Build history of the part. All positions in model axes, mm. A direction names the side the tool comes from. Coordinates: 2 decimals unless noted, no trailing zeros. Loops run counter-clockwise (first coordinate to the right, second up) from the corner with the lowest first, then second, coordinate; pieces in that order, holes last. Notation, with made-up numbers: (79, 56) - (108, 56) arc R29 cw to (108, 77) - close; hole circle Ø1 at (-35, 8). An arc over 180 degrees is marked (long way). One line per item, written item: value.
```python
from build123d import *

# Parameters (mm, degrees)
BOSS_EXTRUDE1_DEPTH = 80
BOSS_EXTRUDE2_DEPTH = 17
SKETCH3_R           = 7.5
CUT_EXTRUDE1_DEPTH  = 17
CUT_EXTRUDE2_DEPTH  = 70
SKETCH6_R           = 6
CUT_EXTRUDE3_DEPTH  = 20


with BuildPart() as part:
    # Sketch1 → Boss-Extrude1 (new body)
    with BuildSketch(Plane.XY):
        Polygon((-12, 17), (-12, -17), (29, -17), (29, -30), (-29, -30), (-29, 30), (29, 30), (29, 17), align=None)
    extrude(amount=-BOSS_EXTRUDE1_DEPTH)

    # Sketch2 → Boss-Extrude2 (add)
    with BuildSketch(Plane.ZY.offset(29)):
        with BuildLine():
            Line((-70, 70.5), (-70, 35.68393157))
            ThreePointArc((-70, 35.68393157), (-71.664785013, 31.664785013), (-75.68393157, 30))
            Line((-75.68393157, 30), (-4.31606843, 30))
            ThreePointArc((-4.31606843, 30), (-8.335214987, 31.664785013), (-10, 35.68393157))
            Line((-10, 35.68393157), (-10, 70.5))
            ThreePointArc((-10, 70.5), (-40, 100.5), (-70, 70.5))
        make_face()
    extrude(amount=-BOSS_EXTRUDE2_DEPTH)

    # Sketch3 → Cut-Extrude1 (cut)
    with BuildSketch(Plane.ZY.offset(29)):
        with Locations(Location((-40, 70.5, 0), (0, 0, 270))):
            Circle(SKETCH3_R)
    extrude(amount=-CUT_EXTRUDE1_DEPTH, mode=Mode.SUBTRACT)

    # Sketch4 → Cut-Extrude2 (cut)
    with BuildSketch(Plane(origin=(0, 30, 0), x_dir=(1, 0, 0), z_dir=(0, 1, 0))):
        with BuildLine():
            Line((9.5, 66), (9.5, 14))
            ThreePointArc((9.5, 14), (16, 7.5), (22.5, 14))
            Line((22.5, 14), (22.5, 66))
            ThreePointArc((22.5, 66), (16, 72.5), (9.5, 66))
        make_face()
    extrude(amount=-CUT_EXTRUDE2_DEPTH, mode=Mode.SUBTRACT)

    # Sketch6 → Cut-Extrude3 (cut)
    with BuildSketch(Plane(origin=(-12, 0, 0), x_dir=(0, 0, -1), z_dir=(1, 0, 0))):
        with Locations(Location((18.5, 0, 0), (0, 0, 90))):
            Circle(SKETCH6_R)
        with Locations(Location((61.5, 0, 0), (0, 0, 90))):
            Circle(SKETCH6_R)
    extrude(amount=-CUT_EXTRUDE3_DEPTH, mode=Mode.SUBTRACT)


solid = part.part
```
Item 1: Cut at D-D, the plane x = -16. Write the cut outline in (y, z).
Check result:
outline: (-30, -80) - (30, -80) - (30, -75.68) arc R5.68 cw to (35.68, -70) - (70.5, -70) arc R30 ccw to (70.5, -10) - (35.68, -10) arc R5.68 cw to (30, -4.32) - (30, 0) - (-30, 0) - close; hole circle Ø12 at (0, -61.5); hole circle Ø12 at (0, -18.5); hole circle Ø15 at (70.5, -40)
Item 2: Cut at A-A, the plane z = -40. Write the cut outline in (x, y).
Check result:
outline: (-29, -30) - (9.5, -30) - (9.5, -17) - (-12, -17) - (-12, 17) - (9.5, 17) - (9.5, 30) - (-12, 30) - (-12, 63) - (-29, 63) - close; (-29, 78) - (-12, 78) - (-12, 100.5) - (-29, 100.5) - close; (22.5, -30) - (29, -30) - (29, -17) - (22.5, -17) - close; (22.5, 17) - (29, 17) - (29, 30) - (22.5, 30) - close
Item 3: Drop flat-ended pins along their axis: P1, Ø24, axis at y = 70.5, z = -40, coming from the -X side; P2, Ø12.5, axis at x = 5, z = -44.5, coming from the +Y side; P3, Ø12, axis at x = -10, y = 61.5, coming from the -Z side; P4, Ø13.5, axis at x = -18, y = 48.5, coming from the +Z side. Give the stop position or say it passes through.
Check result:
P1: stops at x = -29
P2: stops at y = 30
P3: stops at z = -70
P4: stops at z = -10
Item 4: Cut at B-B, the plane x = 13.5. Write the cut outline in (y, z).
Check result:
outline: (-30, -80) - (-17, -80) - (-17, -72) - (-30, -72) - close; (-30, -8) - (-17, -8) - (-17, 0) - (-30, 0) - close; (17, -80) - (30, -80) - (30, -72) - (17, -72) - close; (17, -8) - (30, -8) - (30, 0) - (17, 0) - close
Item 5: Pull direction Y, two halves, no side cores. Call faces 4 (the face through (29, -23, -39)), 5 (the face through (4, 17, -39)), 6 (the face through (-20.381, 5.723, -59.698)), 7 (the face through (-20.62, 31.71, -71.62)): released by +Y, released by -Y, zero draft, split by the parting line, or undercut.
Check result:
face 4: zero draft
face 5: undercut
face 6: undercut
face 7: released by +Y
Item 6: Tool access for faces 1 (the face through (15.9, 23.6, -7.5)), 2 (the face through (-12, 58, -40)), 3 (the face through (-21, 53, -70)): list every direction of +Z, -Z, +X, -X, +Y, -Y with a clear straight run to the whole face (end or side of a thin tool).
Check result:
face 1: +Y, -Y
face 2: +Z, -Z, +X, +Y
face 3: -Z, +X, -X, +Y
Item 7: Probe probe 1 along Z at (x, y) = (-18.5, 0); probe 2 along Y at (x, z) = (-7.5, -49); probe 3 along X at (y, z) = (87, -17). List the from-to ranges inside material, lowest first. Write a range as from..to.
Check result:
probe 1: z = -80..-67.5, -55.5..-24.5, -12.5..0
probe 2: y = -30..-17, 17..30
probe 3: x = -29..-12
Item 8: Cut at C-C, the plane y = 0. Write the cut outline in (x, z), then the cut area to 3 significant figures.
Check result:
outline: (-29, -80) - (-12, -80) - (-12, -67.5) - (-29, -67.5) - close; (-29, -55.5) - (-12, -55.5) - (-12, -24.5) - (-29, -24.5) - close; (-29, -12.5) - (-12, -12.5) - (-12, 0) - (-29, 0) - close
area: 952 mm^2
